Source: CAD feature listing. Evaluate the final solid. Frame: model axes, mm. Coordinates: 2 decimals unless noted, no trailing zeros. Loops run counter-clockwise (first coordinate to the right, second up) from the corner with the lowest first, then second, coordinate; pieces in that order, holes last. Notation, with made-up numbers: M 16,56 L 53,56 A19 cw 53,93 Z; hole C 80,-0.75 d1. An arc over 180 degrees is marked long. Write each question's results on one line, items separated by ' | '. Start each with the question number.
from build123d import *

# Parameters (mm, degrees)
MODEL_R         = 2.054
EXTRUDE_1_DEPTH = 1


with BuildPart() as part:
    # Model → Бобышка-Вытянуть1 (new body)
    with BuildSketch(Plane.XY):
        with BuildLine():
            Line((2635.23603, -2604.35979), (2641.85781, -2604.35979))
            Line((2641.85781, -2604.35979), (2641.85781, -2617.90434))
            Line((2641.85781, -2617.90434), (2661.0288664, -2617.90434))
            ThreePointArc((2661.0288664, -2617.90434), (2661.614235055, -2616.491135055), (2663.02744, -2615.9057664))
            Line((2663.02744, -2615.9057664), (2663.02744, -2567.94))
            Line((2663.02744, -2567.94), (2606.04, -2567.94))
            Line((2606.04, -2567.94), (2606.04, -2615.9137928))
            ThreePointArc((2606.04, -2615.9137928), (2607.447529423, -2616.496810577), (2608.0305472, -2617.90434))
            Line((2608.0305472, -2617.90434), (2635.23603, -2617.90434))
            Line((2635.23603, -2617.90434), (2635.23603, -2604.35979))
        make_face()
        with Locations((2626.50732, -2584.8749456)):
            Circle(MODEL_R, mode=Mode.SUBTRACT)
        with Locations((2659.602587949, -2584.87952199)):
            Circle(MODEL_R, mode=Mode.SUBTRACT)
    extrude(amount=EXTRUDE_1_DEPTH)


solid = part.part
Item 1: Mould query, pull axis X, two halves, no side actions, for faces 1 (the flat face through (2634, -2593, 1)), 2 (the cylindrical face through (2627.455, -2586.697, 0.493)), 3 (the cylindrical face through (2661.599, -2616.507, 0.493)). Classes: +X half, -X half, draft (parallel to the pull), parting line (faces both ways), or undercut.
Item 2: Cut plane A-A (y = -2585.5). Output: boundary loops of the cut face in (x, z).
Item 3: First-contact query: pin 1 Ø2.5 at (x, y) = (2626.51, -2584.87) entering from +Z. Flat tip, straight axial feed; report the tip coordinate or a pass-through.
Item 4: Cut plane B-B (z = 0.15). Output: boundary loops of the cut face in (x, y).
Item 5: Line query: probe 1 along X at (y, z) = (-2611.5, 0.55); probe 2 along Y at (x, z) = (2641.5, 0.25); probe 3 along Y at (x, z) = (2628, 0.85). Output: solid intervals per line, ascending.
Response values:
1) face 1: draft | face 2: undercut | face 3: +X half
2) outline: M 2606.04,0 L 2624.55,0 L 2624.55,1 L 2606.04,1 Z; M 2628.46,0 L 2657.64,0 L 2657.64,1 L 2628.46,1 Z; M 2661.56,0 L 2663.03,0 L 2663.03,1 L 2661.56,1 Z
3) pin 1: passes through
4) outline: M 2606.04,-2615.91 A1.99 cw 2608.03,-2617.9 L 2635.24,-2617.9 L 2635.24,-2604.36 L 2641.86,-2604.36 L 2641.86,-2617.9 L 2661.03,-2617.9 A2 cw 2663.03,-2615.91 L 2663.03,-2567.94 L 2606.04,-2567.94 Z; hole C 2626.51,-2584.87 d4.11; hole C 2659.6,-2584.88 d4.11
5) probe 1: x = 2606.04 to 2635.24, 2641.86 to 2663.03 | probe 2: y = -2604.36 to -2567.94 | probe 3: y = -2617.9 to -2586.29, -2583.46 to -2567.94
